The model under review builds one solid part; all positions refer to its coordinate system, in mm. Coordinates: 2 decimals unless noted, no trailing zeros. Order: outer loops, then holes, each group sorted by start corner. A loop starts at its lowest first (then second) coordinate and runs counter-clockwise, first axis right, second up. Notation, with made-up numbers: M 65,-13.75 L 106,-13.75 A22 ccw 106,22.25 Z; hole C 32,18 d10. An arc over 180 degrees is marked long. Answer as CSV lines item,"result". Start each with the question number.
Q1. Consider section A-A on y = 0. Write out the cut boundary in (x, z), and give its area (3 significant figures).
Q2. Consider section B-B on x = 0.8. State how many separate pieces and enclosed holes the cut face has, and give its area (3 significant figures).
Q3. Consider section D-D on y = 25. Write out the cut boundary in (x, z).
Q4. Wall thickness on L1, parallel to Y at x = 1.3, z = 0; L2, parallel to Y at x = 1, z = 26; L3, parallel to Y at x = 0.9, z = 15: over which ranges is each line inside the solid? List them lowest first. Write a range as [from, to].
Q5. For P1, Ø1.5, axis at x = 1.5, z = 16, coming from the -Y side; P2, Ø2, axis at x = 2, y = -4, coming from the +Z side; P3, Ø2.5, axis at y = -30.5, z = 13.5, coming from the +X side; P4, Ø2, axis at y = 7.25, z = 14, coming from the +X side, all flat-tipped, find the tip position at first contact; note any pin that passes through.
Q6. Consider section C-C on z = 40. Write out the cut boundary in (x, y), and give its area (3 significant figures).
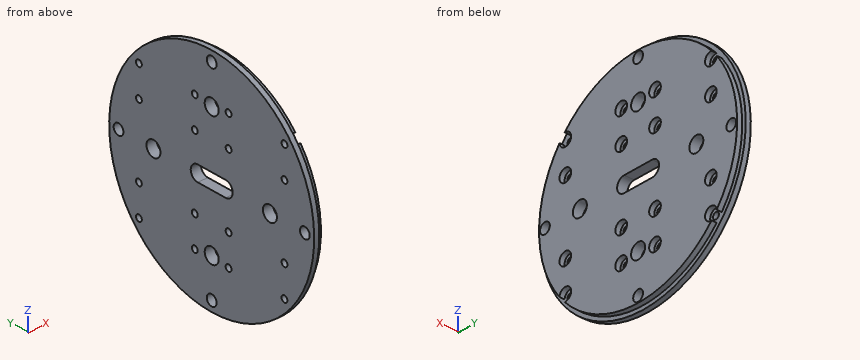
from build123d import *

# Parameters (mm, degrees)
CROQUIS1_R              = 44
SALIENTE_EXTRUIR1_DEPTH = 4
CROQUIS2_R              = 1.25
CORTAR_EXTRUIR2_DEPTH   = 63.353829072
CORTAR_EXTRUIR3_START   = -2
CROQUIS3_R              = 2.5
CORTAR_EXTRUIR3_DEPTH   = 61.353829072
CROQUIS4_R              = 3
CORTAR_EXTRUIR4_DEPTH   = 63.353829072
CROQUIS5_OUTSIDE_W      = 114.904
CROQUIS5_OUTSIDE_H      = 114.904
CROQUIS5_OUTSIDE_R      = 42.5
CORTAR_EXTRUIR5_DEPTH   = 2
CROQUIS6_R              = 2.1
CORTAR_EXTRUIR6_DEPTH   = 63.353829072


with BuildPart() as part:
    # Croquis1 → Saliente-Extruir1 (new body)
    with BuildSketch(Plane(origin=(0, 0, 0), x_dir=(0, 0, -1), z_dir=(1, 0, 0))):
        Circle(CROQUIS1_R)
    extrude(amount=SALIENTE_EXTRUIR1_DEPTH)

    # Croquis2 → Cortar-Extruir2 (cut, through all)
    with BuildSketch(Plane.ZY):
        with Locations((14, 7.25)):
            Circle(CROQUIS2_R)
        with Locations((26, 7.25)):
            Circle(CROQUIS2_R)
        with Locations((26, 31.25)):
            Circle(CROQUIS2_R)
        with Locations((14, 31.25)):
            Circle(CROQUIS2_R)
        with Locations(Location((-26, 31.25, 0), (0, 0, 180))):
            Circle(CROQUIS2_R)
        with Locations(Location((-14, 31.25, 0), (0, 0, 180))):
            Circle(CROQUIS2_R)
        with Locations(Location((-26, 7.25, 0), (0, 0, 180))):
            Circle(CROQUIS2_R)
        with Locations(Location((-14, 7.25, 0), (0, 0, 180))):
            Circle(CROQUIS2_R)
        with Locations((-14, -7.25)):
            Circle(CROQUIS2_R)
        with Locations((-26, -7.25)):
            Circle(CROQUIS2_R)
        with Locations((-14, -31.25)):
            Circle(CROQUIS2_R)
        with Locations((-26, -31.25)):
            Circle(CROQUIS2_R)
        with Locations(Location((14, -31.25, 0), (0, 0, 180))):
            Circle(CROQUIS2_R)
        with Locations(Location((26, -31.25, 0), (0, 0, 180))):
            Circle(CROQUIS2_R)
        with Locations(Location((26, -7.25, 0), (0, 0, 180))):
            Circle(CROQUIS2_R)
        with Locations(Location((14, -7.25, 0), (0, 0, 180))):
            Circle(CROQUIS2_R)
    extrude(amount=-CORTAR_EXTRUIR2_DEPTH, mode=Mode.SUBTRACT)

    # Croquis3 → Cortar-Extruir3 (cut, through all)
    with BuildSketch(Plane.ZY.offset(CORTAR_EXTRUIR3_START)):
        with Locations((14, 7.25)):
            Circle(CROQUIS3_R)
        with Locations((26, 7.25)):
            Circle(CROQUIS3_R)
        with Locations((26, 31.25)):
            Circle(CROQUIS3_R)
        with Locations((14, 31.25)):
            Circle(CROQUIS3_R)
        with Locations(Location((-26, 31.25, 0), (0, 0, 180))):
            Circle(CROQUIS3_R)
        with Locations(Location((-14, 31.25, 0), (0, 0, 180))):
            Circle(CROQUIS3_R)
        with Locations(Location((-26, 7.25, 0), (0, 0, 180))):
            Circle(CROQUIS3_R)
        with Locations(Location((-14, 7.25, 0), (0, 0, 180))):
            Circle(CROQUIS3_R)
        with Locations((-14, -7.25)):
            Circle(CROQUIS3_R)
        with Locations((-26, -7.25)):
            Circle(CROQUIS3_R)
        with Locations((-14, -31.25)):
            Circle(CROQUIS3_R)
        with Locations((-26, -31.25)):
            Circle(CROQUIS3_R)
        with Locations(Location((14, -31.25, 0), (0, 0, 180))):
            Circle(CROQUIS3_R)
        with Locations(Location((26, -31.25, 0), (0, 0, 180))):
            Circle(CROQUIS3_R)
        with Locations(Location((26, -7.25, 0), (0, 0, 180))):
            Circle(CROQUIS3_R)
        with Locations(Location((14, -7.25, 0), (0, 0, 180))):
            Circle(CROQUIS3_R)
    extrude(amount=-CORTAR_EXTRUIR3_DEPTH, mode=Mode.SUBTRACT)

    # Croquis4 → Cortar-Extruir4 (cut, through all)
    with BuildSketch(Plane.ZY):
        with Locations((0, 25)):
            Circle(CROQUIS4_R)
        with Locations((25, 0)):
            Circle(CROQUIS4_R)
        with Locations((0, -25)):
            Circle(CROQUIS4_R)
        with Locations((-25, 0)):
            Circle(CROQUIS4_R)
        with BuildLine():
            Line((3, 6), (3, -6))
            ThreePointArc((3, -6), (0, -9), (-3, -6))
            Line((-3, -6), (-3, 6))
            ThreePointArc((-3, 6), (0, 9), (3, 6))
        make_face()
    extrude(amount=-CORTAR_EXTRUIR4_DEPTH, mode=Mode.SUBTRACT)

    # Croquis5 outside → Cortar-Extruir5 (cut)
    with BuildSketch(Plane(origin=(4, 0, 0), x_dir=(0, 0, -1), z_dir=(1, 0, 0))):
        Rectangle(CROQUIS5_OUTSIDE_W, CROQUIS5_OUTSIDE_H)
        Circle(CROQUIS5_OUTSIDE_R, mode=Mode.SUBTRACT)
    extrude(amount=-CORTAR_EXTRUIR5_DEPTH, mode=Mode.SUBTRACT)

    # Croquis6 → Cortar-Extruir6 (cut, through all)
    with BuildSketch(Plane.ZY):
        with Locations((-40, 0)):
            Circle(CROQUIS6_R)
        with Locations((0, 40)):
            Circle(CROQUIS6_R)
        with Locations((40, 0)):
            Circle(CROQUIS6_R)
        with Locations((0, -40)):
            Circle(CROQUIS6_R)
    extrude(amount=-CORTAR_EXTRUIR6_DEPTH, mode=Mode.SUBTRACT)


solid = part.part
Evaluation:
1,outline,"M 0,-44 L 2,-44 L 2,-42.5 L 4,-42.5 L 4,-42.1 L 0,-42.1 Z; M 0,-37.9 L 4,-37.9 L 4,-28 L 0,-28 Z; M 0,-22 L 4,-22 L 4,-3 L 0,-3 Z; M 0,3 L 4,3 L 4,22 L 0,22 Z; M 0,28 L 4,28 L 4,37.9 L 0,37.9 Z; M 0,42.1 L 4,42.1 L 4,42.5 L 2,42.5 L 2,44 L 0,44 Z"
1,area,"240 mm²"
2,separate pieces,"1"
2,enclosed holes,"25"
2,area,"5,730 mm²"
3,outline,"M 0,-36.21 L 2,-36.21 L 2,-34.37 L 4,-34.37 L 4,-3 L 0,-3 Z; M 0,3 L 4,3 L 4,34.37 L 2,34.37 L 2,36.21 L 0,36.21 Z"
4,L1,"y = [-44, -42.1], [-37.9, -28], [-22, -9], [9, 22], [28, 37.9], [42.1, 44]"
4,L2,"y = [-35.5, -32.5], [-30, -8.5], [-6, -2.83], [2.83, 6], [8.5, 30], [32.5, 35.5]"
4,L3,"y = [-41.36, -32], [-30.5, -8], [-6.5, 6.5], [8, 30.5], [32, 41.36]"
5,P1,"stops at y = -41.27"
5,P2,"stops at z = 43.9"
5,P3,"stops at x = 2"
5,P4,"passes through"
6,outline,"M 0,-18.33 L 2,-18.33 L 2,-14.36 L 4,-14.36 L 4,-2.1 L 0,-2.1 Z; M 0,2.1 L 4,2.1 L 4,14.36 L 2,14.36 L 2,18.33 L 0,18.33 Z"
6,area,"114 mm²"
